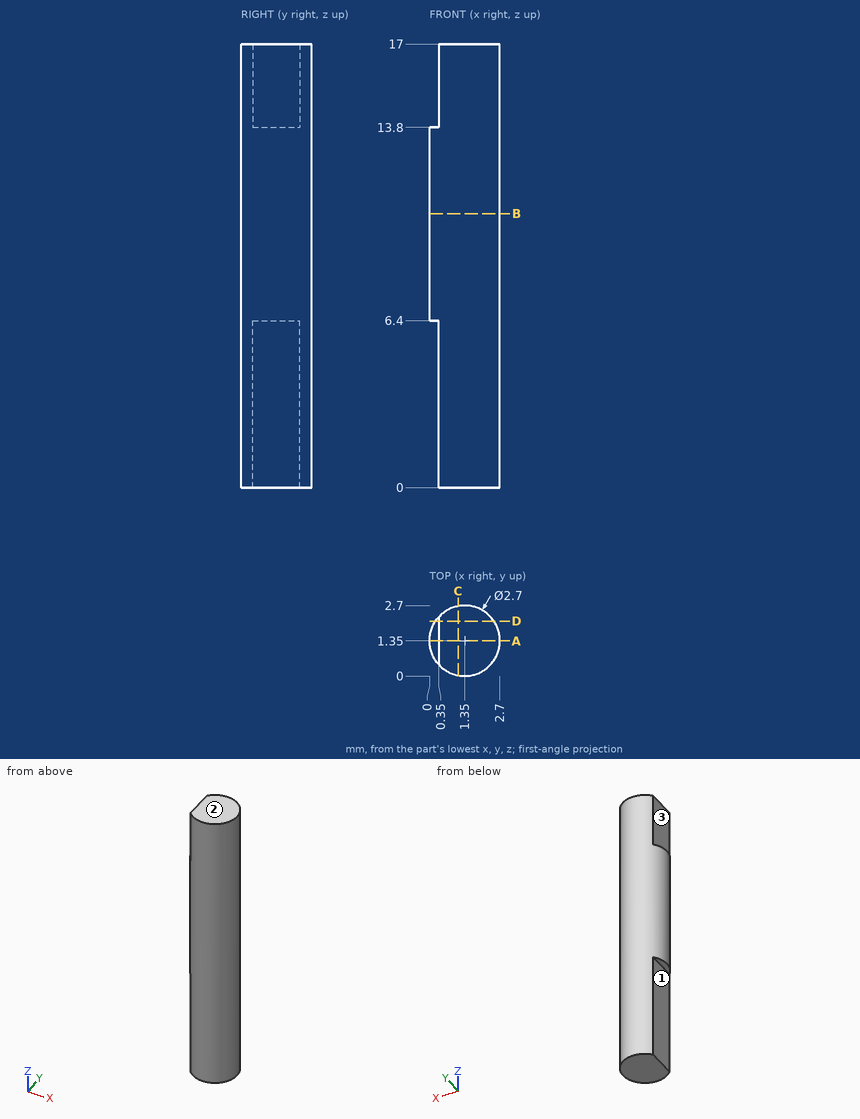
Answer from the drawing. Dimensions are ordinates in mm from the lowest x, y and z of the part. A direction names the side the tool comes from. Give positions to 0.01 mm unless a question says otherwise; leave off trailing zeros. Order: outer loops, then holes, each group sorted by start corner. A loop starts at its lowest first (then second) coordinate and runs counter-clockwise, first axis right, second up. Notation, with made-up numbers: (58, 33) - (65, 33) arc R14 ccw to (65, 53) - close; hole circle Ø7 at (69, -27). An arc over 180 degrees is marked (long way). Use one line per item in the form item = value.
1) Find section D-D on y = 2.1. Determine the outline of the cut face in (x, z), and give its area (3 significant figures).
Verdict:
outline = (0.23, 6.4) - (0.35, 6.4) - (0.35, 0) - (2.47, 0) - (2.47, 17) - (0.35, 17) - (0.35, 13.8) - (0.23, 13.8) - close
area = 37.0 mm^2
2) Each of these flat-tipped pins is pushed along its axis until it touches: pin 1 (1 mm diameter, centred on x = 1, z = 13.5, fed in from -Y); pin 2 (1.5 mm diameter, centred on y = 1, z = 15.5, fed in from -X). Where does it stop, or does it pass through?
Verdict:
pin_1 = 0
pin_2 = 0.35
3) Consider probe 1 along Y at (x, z) = (1.4, 15.75); probe 2 along X at (y, z) = (0.35, 15); probe 3 along Y at (x, z) = (2.05, 10.5). Determine where each line is inside the solid, lowest interval first. Write a range as [from, to].
Verdict:
probe_1 = [0, 2.7]
probe_2 = [0.44, 2.26]
probe_3 = [0.2, 2.5]
4) For the marked faces 1, 2 and 3, determine the directions among +Z, -Z, +X, -X, +Y, -Y from which every point of the face is accessible in a straight line to the end or side of a thin tool.
Verdict:
face_1 = -Z, -X, +Y, -Y
face_2 = +Z, +X, -X, +Y, -Y
face_3 = +Z, -X, +Y, -Y
5) Find section B-B on z = 10.5. Determine the outline of the cut face in (x, y).
Verdict:
outline = circle Ø2.7 at (1.35, 1.35)
6) Find section C-C on x = 1.1. Determine the outline of the cut face in (y, z), and give its area (3 significant figures).
Verdict:
outline = (0.02, 0) - (2.68, 0) - (2.68, 17) - (0.02, 17) - close
area = 45.1 mm^2
7) Find section A-A on y = 1.35. Determine the outline of the cut face in (x, z).
Verdict:
outline = (0, 6.4) - (0.35, 6.4) - (0.35, 0) - (2.7, 0) - (2.7, 17) - (0.35, 17) - (0.35, 13.8) - (0, 13.8) - close
